from build123d import *

# Parameters (mm, degrees)
SKETCH1_R           = 33.325
BOSS_EXTRUDE1_DEPTH = 3


with BuildPart() as part:
    # Sketch1 → Boss-Extrude1 (new body)
    with BuildSketch(Plane(origin=(0, 0, 0), x_dir=(1, 0, 0), z_dir=(0, 1, 0))):
        with Locations(Location((0, 0, 0), (0, 0, 270))):
            Circle(SKETCH1_R)
        with BuildLine():
            Line((1.755453897, 1), (1.755453897, 31.275773477))
            ThreePointArc((1.755453897, 31.275773477), (0, 31.325), (-1.755453897, 31.275773477))
            Line((-1.755453897, 31.275773477), (-1.755453897, 1))
            Line((-1.755453897, 1), (1.755453897, 1))
        make_face(mode=Mode.SUBTRACT)
        with BuildLine():
            Line((29.30999287, 1), (29.30999287, 11.053503651))
            ThreePointArc((29.30999287, 11.053503651), (27.758242919, 14.516734311), (25.799085075, 17.766902776))
            Line((25.799085075, 17.766902776), (25.799085075, 1))
            Line((25.799085075, 1), (29.30999287, 1))
        make_face(mode=Mode.SUBTRACT)
        with BuildLine():
            Line((3.755453897, 1), (7.266361692, 1))
            Line((7.266361692, 1), (7.266361692, 30.470569617))
            ThreePointArc((7.266361692, 30.470569617), (5.519860332, 30.834830418), (3.755453897, 31.099070581))
            Line((3.755453897, 31.099070581), (3.755453897, 1))
        make_face(mode=Mode.SUBTRACT)
        with BuildLine():
            Line((9.266361692, 1), (12.777269486, 1))
            Line((12.777269486, 1), (12.777269486, 28.600647011))
            ThreePointArc((12.777269486, 28.600647011), (11.041631222, 29.314467502), (9.266361692, 29.923070798))
            Line((9.266361692, 29.923070798), (9.266361692, 1))
        make_face(mode=Mode.SUBTRACT)
        with BuildLine():
            Line((14.777269486, 1), (18.288177281, 1))
            Line((18.288177281, 1), (18.288177281, 25.432227522))
            ThreePointArc((18.288177281, 25.432227522), (16.568886372, 26.584349332), (14.777269486, 27.620425984))
            Line((14.777269486, 27.620425984), (14.777269486, 1))
        make_face(mode=Mode.SUBTRACT)
        with BuildLine():
            Line((20.288177281, 1), (23.799085075, 1))
            Line((23.799085075, 1), (23.799085075, 20.36809207))
            ThreePointArc((23.799085075, 20.36809207), (22.112953153, 22.187224429), (20.288177281, 23.867247173))
            Line((20.288177281, 23.867247173), (20.288177281, 1))
        make_face(mode=Mode.SUBTRACT)
        with BuildLine():
            Line((1, -3.570162886), (1, -1))
            Line((1, -1), (3.570162886, -1))
            Line((3.570162886, -1), (17.853404495, -25.739300164))
            ThreePointArc((17.853404495, -25.739300164), (16.382380994, -26.699685728), (14.859831538, -27.576095294))
            Line((14.859831538, -27.576095294), (1, -3.570162886))
        make_face(mode=Mode.SUBTRACT)
        with BuildLine():
            Line((5.879563963, -1), (19.469969491, -24.53927287))
            ThreePointArc((19.469969491, -24.53927287), (20.842468862, -23.384762491), (22.146644648, -22.153594648))
            Line((22.146644648, -22.153594648), (9.933611084, -1))
            Line((9.933611084, -1), (5.879563963, -1))
        make_face(mode=Mode.SUBTRACT)
        with BuildLine():
            Line((12.24301216, -1), (23.574814489, -20.627257375))
            ThreePointArc((23.574814489, -20.627257375), (24.780818594, -19.161593223), (25.895841507, -17.625578506))
            Line((25.895841507, -17.625578506), (16.297059281, -1))
            Line((16.297059281, -1), (12.24301216, -1))
        make_face(mode=Mode.SUBTRACT)
        with BuildLine():
            Line((18.606460358, -1), (27.100022956, -15.711281958))
            ThreePointArc((27.100022956, -15.711281958), (28.097453336, -13.848781211), (28.967067125, -11.923281729))
            Line((28.967067125, -11.923281729), (22.660507478, -1))
            Line((22.660507478, -1), (18.606460358, -1))
        make_face(mode=Mode.SUBTRACT)
        with BuildLine():
            Line((24.969908555, -1), (29.85953815, -9.469086888))
            ThreePointArc((29.85953815, -9.469086888), (30.538044757, -6.977352466), (31.0089993, -4.438196413))
            Line((31.0089993, -4.438196413), (29.023955676, -1))
            Line((29.023955676, -1), (24.969908555, -1))
        make_face(mode=Mode.SUBTRACT)
        with BuildLine():
            Line((1, -7.570162886), (13.066371144, -28.46973077))
            ThreePointArc((13.066371144, -28.46973077), (11.431797975, -29.164526742), (9.760473509, -29.765563692))
            Line((9.760473509, -29.765563692), (1, -14.591978475))
            Line((1, -14.591978475), (1, -7.570162886))
        make_face(mode=Mode.SUBTRACT)
        with BuildLine():
            Line((1, -18.591978475), (7.784125884, -30.342429191))
            ThreePointArc((7.784125884, -30.342429191), (5.971968683, -30.750466908), (4.138812131, -31.050376151))
            Line((4.138812131, -31.050376151), (1, -25.613794064))
            Line((1, -25.613794064), (1, -18.591978475))
        make_face(mode=Mode.SUBTRACT)
        with BuildLine():
            Line((-29.30999287, 1), (-25.799085075, 1))
            Line((-25.799085075, 1), (-25.799085075, 17.766902776))
            ThreePointArc((-25.799085075, 17.766902776), (-27.758242919, 14.516734311), (-29.30999287, 11.053503651))
            Line((-29.30999287, 11.053503651), (-29.30999287, 1))
        make_face(mode=Mode.SUBTRACT)
        with BuildLine():
            Line((-20.288177281, 1), (-23.799085075, 1))
            Line((-23.799085075, 1), (-23.799085075, 20.36809207))
            ThreePointArc((-23.799085075, 20.36809207), (-22.112953153, 22.187224429), (-20.288177281, 23.867247173))
            Line((-20.288177281, 23.867247173), (-20.288177281, 1))
        make_face(mode=Mode.SUBTRACT)
        with BuildLine():
            Line((-14.777269486, 1), (-18.288177281, 1))
            Line((-18.288177281, 1), (-18.288177281, 25.432227522))
            ThreePointArc((-18.288177281, 25.432227522), (-16.568886372, 26.584349332), (-14.777269486, 27.620425984))
            Line((-14.777269486, 27.620425984), (-14.777269486, 1))
        make_face(mode=Mode.SUBTRACT)
        with BuildLine():
            Line((-9.266361692, 1), (-12.777269486, 1))
            Line((-12.777269486, 1), (-12.777269486, 28.600647011))
            ThreePointArc((-12.777269486, 28.600647011), (-11.041631222, 29.314467502), (-9.266361692, 29.923070798))
            Line((-9.266361692, 29.923070798), (-9.266361692, 1))
        make_face(mode=Mode.SUBTRACT)
        with BuildLine():
            Line((-3.755453897, 1), (-7.266361692, 1))
            Line((-7.266361692, 1), (-7.266361692, 30.470569617))
            ThreePointArc((-7.266361692, 30.470569617), (-5.519860332, 30.834830418), (-3.755453897, 31.099070581))
            Line((-3.755453897, 31.099070581), (-3.755453897, 1))
        make_face(mode=Mode.SUBTRACT)
        with BuildLine():
            Line((-24.969908555, -1), (-29.023955676, -1))
            Line((-29.023955676, -1), (-31.0089993, -4.438196413))
            ThreePointArc((-31.0089993, -4.438196413), (-30.538044757, -6.977352466), (-29.85953815, -9.469086888))
            Line((-29.85953815, -9.469086888), (-24.969908555, -1))
        make_face(mode=Mode.SUBTRACT)
        with BuildLine():
            Line((-18.606460358, -1), (-22.660507478, -1))
            Line((-22.660507478, -1), (-28.967067125, -11.923281729))
            ThreePointArc((-28.967067125, -11.923281729), (-28.097453336, -13.848781211), (-27.100022956, -15.711281958))
            Line((-27.100022956, -15.711281958), (-18.606460358, -1))
        make_face(mode=Mode.SUBTRACT)
        with BuildLine():
            Line((-12.24301216, -1), (-16.297059281, -1))
            Line((-16.297059281, -1), (-25.895841507, -17.625578506))
            ThreePointArc((-25.895841507, -17.625578506), (-24.780818594, -19.161593223), (-23.574814489, -20.627257375))
            Line((-23.574814489, -20.627257375), (-12.24301216, -1))
        make_face(mode=Mode.SUBTRACT)
        with BuildLine():
            Line((-5.879563963, -1), (-9.933611084, -1))
            Line((-9.933611084, -1), (-22.146644648, -22.153594648))
            ThreePointArc((-22.146644648, -22.153594648), (-20.842468862, -23.384762491), (-19.469969491, -24.53927287))
            Line((-19.469969491, -24.53927287), (-5.879563963, -1))
        make_face(mode=Mode.SUBTRACT)
        with BuildLine():
            Line((-1, -1), (-3.570162886, -1))
            Line((-3.570162886, -1), (-17.853404495, -25.739300164))
            ThreePointArc((-17.853404495, -25.739300164), (-16.382380994, -26.699685728), (-14.859831538, -27.576095294))
            Line((-14.859831538, -27.576095294), (-1, -3.570162886))
            Line((-1, -3.570162886), (-1, -1))
        make_face(mode=Mode.SUBTRACT)
        with BuildLine():
            Line((-1, -7.570162886), (-1, -14.591978475))
            Line((-1, -14.591978475), (-9.760473509, -29.765563692))
            ThreePointArc((-9.760473509, -29.765563692), (-11.431797975, -29.164526742), (-13.066371144, -28.46973077))
            Line((-13.066371144, -28.46973077), (-1, -7.570162886))
        make_face(mode=Mode.SUBTRACT)
        with BuildLine():
            Line((-1, -18.591978475), (-1, -25.613794064))
            Line((-1, -25.613794064), (-4.138812131, -31.050376151))
            ThreePointArc((-4.138812131, -31.050376151), (-5.971968683, -30.750466908), (-7.784125884, -30.342429191))
            Line((-7.784125884, -30.342429191), (-1, -18.591978475))
        make_face(mode=Mode.SUBTRACT)
    extrude(amount=BOSS_EXTRUDE1_DEPTH)


solid = part.part
For this review, take the finished solid that the model builds, in its own axes (mm). Round coordinates to 2 decimals unless told otherwise and drop trailing zeros. Order: outer loops, then holes, each group sorted by start corner. A loop starts at its lowest first (then second) coordinate and runs counter-clockwise, first axis right, second up. Notation, with made-up numbers: M 56.25,53 L 97.25,53 A27 cw 97.25,80 Z; hole C 54,81.25 d1. An arc over 180 degrees is marked long. Use a Markdown table: item, result. Add a question column.
Item 1: Insertion check: pin 1 (1.5 mm diameter, centred on y = 2, z = -9, fed in from +X); pin 2 (0.9 mm diameter, centred on y = 1.5, z = -6.5, fed in from -X); pin 3 (1.5 mm diameter, centred on x = 7, y = 1.5, fed in from +Z). Each pin has a flat end and moves straight along its axis. Give the tip position at first contact, or say it passes through.
Item 2: Mouldability with a two-part tool opening along Z and no side actions: class faces 1 (the flat face through (21.164, 1.479, 9.429)), 2 (the flat face through (25.86, 1.48, 6.54)) as released by +Z, released by -Z, zero draft, split by the parting line, or undercut.
Item 3: Add section A-A, the plane x = 0. Give the boundary of the cut face in (y, z) (3 decimals), then the cut area to 3 significant figures.
Item 4: Add section B-B, the plane y = 0.45. State how many separate pieces and enclosed holes the cut face has, then the cut area to 3 significant figures.
Item 5: To check wall thickness, follow line 1 along Z through (x, y) = (-0.5, 2.7); line 2 along Z through (x, y) = (-10.5, 2.6); line 3 along Z through (x, y) = (-9, 2.7). State the ranges of each line that lie inside material, in increasing order.
Geometry results:
| question | item | result |
|---|---|---|
| 1 | pin 1 | stops at x = 32.29 |
| 1 | pin 2 | stops at x = -32.77 |
| 1 | pin 3 | stops at z = 32.73 |
| 2 | face 1 | undercut |
| 2 | face 2 | undercut |
| 3 | outline | M 0,-33.325 L 3,-33.325 L 3,-31.325 L 0,-31.325 Z; M 0,-1 L 3,-1 L 3,33.325 L 0,33.325 Z |
| 3 | area | 109 mm² |
| 4 | separate pieces | 1 |
| 4 | enclosed holes | 25 |
| 4 | area | 1,650 mm² |
| 5 | line 1 | z = -33.32 to -31.32, -1 to 33.32 |
| 5 | line 2 | z = -31.63 to -29.51, -1 to 1.98, 9 to 13, 20.02 to 24.02, 29.51 to 31.63 |
| 5 | line 3 | z = -32.09 to 1, 6.4 to 10.4, 17.43 to 21.43, 28.45 to 32.09 |
